Check sheet for the modelled part. Datum: model origin and axes. Units: mm. Face numbers are marked on the shaded views. A direction names the side the tool comes from. Give positions to 0.01 mm unless a question says otherwise; leave off trailing zeros. Order: outer loops, then holes, each group sorted by start corner. A loop starts at its lowest first (then second) coordinate and runs counter-clockwise, first axis right, second up.
Item 1: Sectioned sample at B-B on x = 10. Record the boundary of the cut face in (y, z), and give its area (3 significant figures).
Item 2: Gauge pin test, flat ends, axial feed: P1, Ø1.2, axis at x = 52.5, y = 32, coming from the +Z side; P2, Ø15.5, axis at y = 13, z = 26.5, coming from the -X side; P3, Ø5, axis at x = 15.5, y = 27, coming from the +Z side. Record the tip position at first contact, or that the pin passes through.
Item 3: Sectioned sample at C-C on z = 13. Record the boundary of the cut face in (x, y), and give its area (3 significant figures).
Item 4: Sectioned sample at A-A on y = 18. Record the boundary of the cut face in (x, z).
Item 5: Access from +Z, -Z, +X, -X, +Y, -Y to the whole of each face (thin tool, end or side, straight path). Record for the marked faces 5, 6 and 7.
Item 6: Release check for a two-part mould opening along X. For the marked faces 1, 2, 3 and 4 record: released by +X, released by -X, zero draft, split by the parting line, or undercut.
Item 7: Sectioned sample at D-D on y = 14. Record the boundary of the cut face in (x, z).
Item 8: Material ranges on line 1 along X through (y, z) = (22, 27.5); line 2 along Y through (x, z) = (10, 2); line 3 along Y through (x, z) = (44.5, 9.5), recorded low to high.
from build123d import *

# Parameters (mm, degrees)
SKETCH_W        = 56
SKETCH_H        = 36
PAD_DEPTH       = 5
SKETCH001_W     = 21
SKETCH001_H     = 36
PAD001_DEPTH    = 30
SKETCH002_W     = 16
SKETCH002_H     = 31
POCKET_DEPTH    = 33
SKETCH003_R     = 2.45
PAD002_DEPTH    = 30.5
SKETCH004_W     = 3.5
SKETCH004_H     = 6.5
POCKET001_DEPTH = 2
SKETCH005_R     = 2
POCKET002_DEPTH = 5


with BuildPart() as part:
    # Sketch → Pad (new body)
    with BuildSketch(Plane.XY):
        with Locations((28, 18)):
            Rectangle(SKETCH_W, SKETCH_H)
    extrude(amount=PAD_DEPTH)

    # Sketch001 (on Face6 of Pad) → Pad001 (join)
    with BuildSketch(Plane.XY.offset(5)):
        with Locations((45.5, 18)):
            Rectangle(SKETCH001_W, SKETCH001_H)
    extrude(amount=PAD001_DEPTH)

    # Sketch002 (on Face10 of Pad001) → Pocket (cut)
    with BuildSketch(Plane.XY.offset(35)):
        with Locations((45.5, 18)):
            Rectangle(SKETCH002_W, SKETCH002_H)
    extrude(amount=-POCKET_DEPTH, mode=Mode.SUBTRACT)

    # Sketch003 (on Face16 of Pocket) → Pad002 (join)
    with BuildSketch(Plane.XY.offset(2)):
        with Locations((37.5, 33.5)):
            Circle(SKETCH003_R)
        with Locations((53.5, 33.5)):
            Circle(SKETCH003_R)
        with Locations((37.5, 2.5)):
            Circle(SKETCH003_R)
        with Locations((53.5, 2.5)):
            Circle(SKETCH003_R)
    extrude(amount=PAD002_DEPTH)

    # Sketch004 (on Face18 of Pad002) → Pocket001 (cut)
    with BuildSketch(Plane.XY.offset(2)):
        with Locations((45.513299, 17.941233)):
            Rectangle(SKETCH004_W, SKETCH004_H)
    extrude(amount=-POCKET001_DEPTH, mode=Mode.SUBTRACT)

    # Sketch005 (on Face5 of Pocket001) → Pocket002 (cut)
    with BuildSketch(Plane.XY.offset(5)):
        with Locations((10, 18)):
            Circle(SKETCH005_R)
    extrude(amount=-POCKET002_DEPTH, mode=Mode.SUBTRACT)


solid = part.part
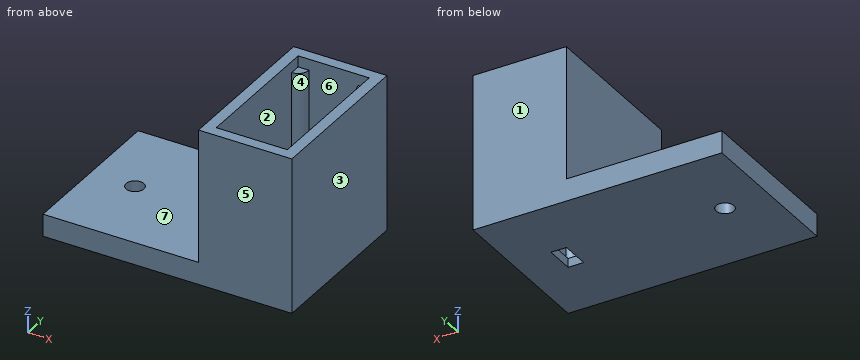
Report:
1. outline: (0, 0) - (16, 0) - (16, 5) - (0, 5) - close; (20, 0) - (36, 0) - (36, 5) - (20, 5) - close
1. area: 160 mm2
2. P1: stops at z = 32.5
2. P2: stops at x = 35
2. P3: stops at z = 5
3. outline: (35, 0) - (56, 0) - (56, 36) - (35, 36) - close; hole (37.5, 4.95) arc R2.45 cw to (39.95, 2.5) - (51.05, 2.5) arc R2.45 cw to (53.5, 4.95) - (53.5, 31.05) arc R2.45 cw to (51.05, 33.5) - (39.95, 33.5) arc R2.45 cw to (37.5, 31.05) - close
3. area: 279 mm2
4. outline: (0, 0) - (8, 0) - (8, 5) - (0, 5) - close; (12, 0) - (43.76, 0) - (43.76, 2) - (37.5, 2) - (37.5, 35) - (35, 35) - (35, 5) - (12, 5) - close; (47.26, 0) - (56, 0) - (56, 35) - (53.5, 35) - (53.5, 2) - (47.26, 2) - close
5. face 5: +Z, -Z, +X, -X, -Y
5. face 6: +Z
5. face 7: +Z, -X, +Y, -Y
6. face 1: zero draft
6. face 2: undercut
6. face 3: released by +X
6. face 4: undercut
7. outline: (0, 0) - (56, 0) - (56, 35) - (53.5, 35) - (53.5, 2) - (37.5, 2) - (37.5, 35) - (35, 35) - (35, 5) - (0, 5) - close
8. line 1: x = 35 to 37.5, 53.5 to 56
8. line 2: y = 0 to 16, 20 to 36
8. line 3: y = 0 to 2.5, 33.5 to 36
